```python
from build123d import *

# Parameters (mm, degrees)
SKETCH1_R               = 1.6
BOSS_EXTRUDE1_DEPTH     = 6
SKETCH5_W               = 262
SKETCH5_H               = 6
BOSS_EXTRUDE3_DEPTH     = 40
SKETCH5_2_W             = 262
SKETCH5_2_H             = 6
BOSS_EXTRUDE5_DEPTH     = 30
SKETCH3_R               = 2.1
CUT_EXTRUDE1_DEPTH      = 189.164821367
SKETCH6_W               = 225
SKETCH6_H               = 77
CUT_EXTRUDE2_DEPTH      = 153.47950682
BOSS_EXTRUDE7_DEPTH     = 20
CUT_EXTRUDE4_DEPTH      = 189.164821367
CUT_EXTRUDE4_DEPTH_BACK = 189.164821367
SKETCH11_W              = 36
SKETCH11_H              = 9
SKETCH11_W_2            = 13.5
SKETCH11_H_2            = 25
SKETCH11_W_3            = 205
BOSS_EXTRUDE4_DEPTH     = 3
BOSS_EXTRUDE6_DEPTH     = 3
FILLET1_R               = 2


with BuildPart() as part:
    # Sketch1 → Boss-Extrude1 (new body)
    with BuildSketch(Plane.XY):
        Polygon((-131, -66), (-131, 66), (131, 66), (131, -66), (131, -67), (-131, -67), align=None)
        with Locations((-121, 56)):
            Circle(SKETCH1_R, mode=Mode.SUBTRACT)
        with Locations((121, 56)):
            Circle(SKETCH1_R, mode=Mode.SUBTRACT)
        with Locations((121, -56)):
            Circle(SKETCH1_R, mode=Mode.SUBTRACT)
        with Locations((-121, -56)):
            Circle(SKETCH1_R, mode=Mode.SUBTRACT)
    extrude(amount=BOSS_EXTRUDE1_DEPTH)

    # Sketch5 → Boss-Extrude3 (add)
    with BuildSketch(Plane.XY.offset(6)):
        with Locations((0, -64)):
            Rectangle(SKETCH5_W, SKETCH5_H)
    extrude(amount=BOSS_EXTRUDE3_DEPTH)

    # Sketch5<2> → Boss-Extrude5 (add)
    with BuildSketch(Plane.XY.offset(6)):
        with Locations((0, -64)):
            Rectangle(SKETCH5_2_W, SKETCH5_2_H)
    extrude(amount=-BOSS_EXTRUDE5_DEPTH)

    # Sketch3 → Cut-Extrude1 (cut, through all)
    with BuildSketch(Plane(origin=(0, -61, 0), x_dir=(1, 0, 0), z_dir=(0, 1, 0))):
        with Locations(Location((-110, -41, 0), (0, 0, 270))):
            Circle(SKETCH3_R)
        with Locations(Location((110, -41, 0), (0, 0, 270))):
            Circle(SKETCH3_R)
        with Locations(Location((-90, 19, 0), (0, 0, 270))):
            Circle(SKETCH3_R)
        with Locations(Location((90, 19, 0), (0, 0, 270))):
            Circle(SKETCH3_R)
    extrude(amount=-CUT_EXTRUDE1_DEPTH, mode=Mode.SUBTRACT)

    # Sketch6 → Cut-Extrude2 (cut, through all)
    with BuildSketch(Plane.XY.offset(6)):
        with Locations((0, 27.5)):
            Rectangle(SKETCH6_W, SKETCH6_H)
    extrude(amount=-CUT_EXTRUDE2_DEPTH, mode=Mode.SUBTRACT)

    # Sketch9 → Boss-Extrude7 (add)
    with BuildSketch(Plane(origin=(0, -61, 0), x_dir=(1, 0, 0), z_dir=(0, 1, 0))):
        Polygon((-81.5, 24), (-81.5, 0), (-77.5, 0), (-77.5, 20), (-57.5, 20), (-57.5, 24), align=None)
        Polygon((77.5, 20), (77.5, 0), (81.5, 0), (81.5, 24), (57.5, 24), (57.5, 20), align=None)
    extrude(amount=BOSS_EXTRUDE7_DEPTH)

    # Sketch11 → Cut-Extrude4 (cut, two sides: drawn at the far end of the back side and taken through both)
    with BuildSketch(Plane(origin=(0, -61, 0), x_dir=(1, 0, 0), z_dir=(0, 1, 0)).offset(-CUT_EXTRUDE4_DEPTH_BACK)):
        with Locations((-113, 19.5)):
            Rectangle(SKETCH11_W, SKETCH11_H)
        with Locations((113, 19.5)):
            Rectangle(SKETCH11_W, SKETCH11_H)
        with Locations((124.25, -33.5)):
            Rectangle(SKETCH11_W_2, SKETCH11_H_2)
        with Locations((-124.25, -33.5)):
            Rectangle(SKETCH11_W_2, SKETCH11_H_2)
        with Locations((0, -33.5)):
            Rectangle(SKETCH11_W_3, SKETCH11_H_2)
    extrude(amount=CUT_EXTRUDE4_DEPTH + CUT_EXTRUDE4_DEPTH_BACK, mode=Mode.SUBTRACT)

    # Sketch8 → Boss-Extrude4 (add)
    with BuildSketch(Plane(origin=(131, 0, 0), x_dir=(0, 0, -1), z_dir=(1, 0, 0))):
        Polygon((-6, 66), (-21, -61), (-6, -61), align=None)
        Polygon((0, 66), (0, -61), (15, -61), align=None)
    extrude(amount=-BOSS_EXTRUDE4_DEPTH)

    # Sketch7 → Boss-Extrude6 (add)
    with BuildSketch(Plane.ZY.offset(131)):
        Polygon((6, 66), (21, -61), (6, -61), align=None)
        Polygon((0, 66), (-15, -61), (0, -61), align=None)
    extrude(amount=-BOSS_EXTRUDE6_DEPTH)

    # Fillet1
    fillet1_edges = [part.edges().sort_by_distance(p)[0] for p in [
        (128, 2.5, 6),
        (128, 2.5, 0),
        (-128, 2.5, 0),
        (-131, 2.5, -7.5),
        (-131, 2.5, 13.5),
        (-128, 2.5, 6),
        (131, 2.5, -7.5),
        (131, 2.5, 13.5),
        (-112.5, 27.5, 6),
        (-112.5, 27.5, 0),
        (112.5, 27.5, 6),
        (112.5, 27.5, 0),
        (-131, -64, -15),
        (-95, -64, -15),
        (-95, -64, -24),
        (-81.5, -51, 0),
        (81.5, -51, 0),
        (95, -64, -24),
        (95, -64, -15),
        (131, -64, -15),
        (-131, -64, 21),
        (-117.5, -64, 21),
        (102.5, -64, 21),
        (131, -64, 21),
        (-102.5, -64, 21),
        (117.5, -64, 21),
        (102.5, -64, 46),
        (117.5, -64, 46),
        (-117.5, -64, 46),
        (-102.5, -64, 46),
        (77.5, -51, 0),
        (-77.5, -51, 0),
        (-77.5, -51, -20),
        (77.5, -51, -20),
        (57.5, -51, -20),
        (-57.5, -51, -20),
        (-81.5, -51, -24),
        (-57.5, -51, -24),
        (57.5, -51, -24),
        (81.5, -51, -24),
    ]]
    fillet(fillet1_edges, radius=FILLET1_R - 0.0001)  # a hair under: the kernel refuses the full size


solid = part.part
```
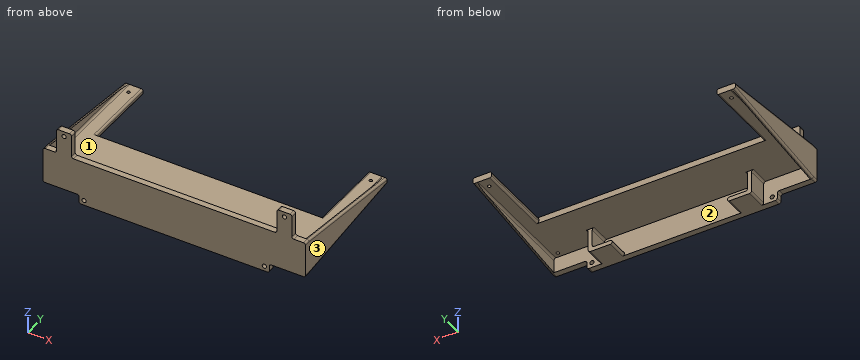
Design review of the part built by this model. Coordinates are the model's own, in mm. Face numbers are marked on the shaded views. A direction names the side the tool comes from. Give positions to 0.01 mm unless a question says otherwise; leave off trailing zeros. Loops run counter-clockwise (first coordinate to the right, second up) from the corner with the lowest first, then second, coordinate; pieces in that order, holes last. Notation, with made-up numbers: (-23.5, 73) -> (-11.5, 73) arc R21 cw to (-11.5, 90) -> close; hole circle Ø2 at (35, 53.25). An arc over 180 degrees is marked (long way). One line per item, written item: value.
Q1. Machinability: for the marked faces 1, 2 and 3, which of the approach directions +Z, -Z, +X, -X, +Y, -Y give a long, thin tool a straight path to every point of the face, cutting with its end or side? Answer none if there is none.
Numbers:
face 1: +Z, +Y
face 2: +Y
face 3: +Z, -Z, +X, +Y, -Y
Q2. For pin 1 Ø1.5 at (x, z) = (-19, 7) entering from +Y; pin 2 Ø6.5 at (y, z) = (-63.5, 32) entering from +X; pin 3 Ø5 at (x, y) = (64, -47.5) entering from +Z, all flat-tipped, find the tip position at first contact; note any pin that passes through.
Numbers:
pin 1: stops at y = -61
pin 2: stops at x = 117.5
pin 3: stops at z = 6
Q3. We need section A-A on x = -50. Give the boundary of the cut face in (y, z).
Numbers:
outline: (-67, -24) -> (-61, -24) -> (-61, 0) -> (-11, 0) -> (-11, 6) -> (-61, 6) -> (-61, 21) -> (-67, 21) -> close
Q4. For L1, parallel to X at y = -64.75, z = -19; L2, parallel to X at y = -64.45, z = 41; L3, parallel to Y at x = -121, z = 2, list the stretches that pass through material, from the lowest coordinate up.
Numbers:
L1: x = -95 to -92.1, -87.9 to 87.9, 92.1 to 95
L2: x = -117.5 to -112.1, -107.9 to -102.5, 102.5 to 107.9, 112.1 to 117.5
L3: y = -67 to -57.6, -54.4 to 54.4, 57.6 to 66
